Geometry check sheet. Reference: drawing and pictorial views, mm from the part's lowest x, y, z. Coordinates: 2 decimals unless noted, no trailing zeros. Loops run counter-clockwise (first coordinate to the right, second up) from the corner with the lowest first, then second, coordinate; pieces in that order, holes last. Notation, with made-up numbers: M -33.75,-31.5 L -20.75,-31.5 A7 ccw -20.75,-20.5 Z; hole C 50,-39 d3. An arc over 180 degrees is marked long. Write each question's results on one line, items separated by ' | '. Start each with the question number.
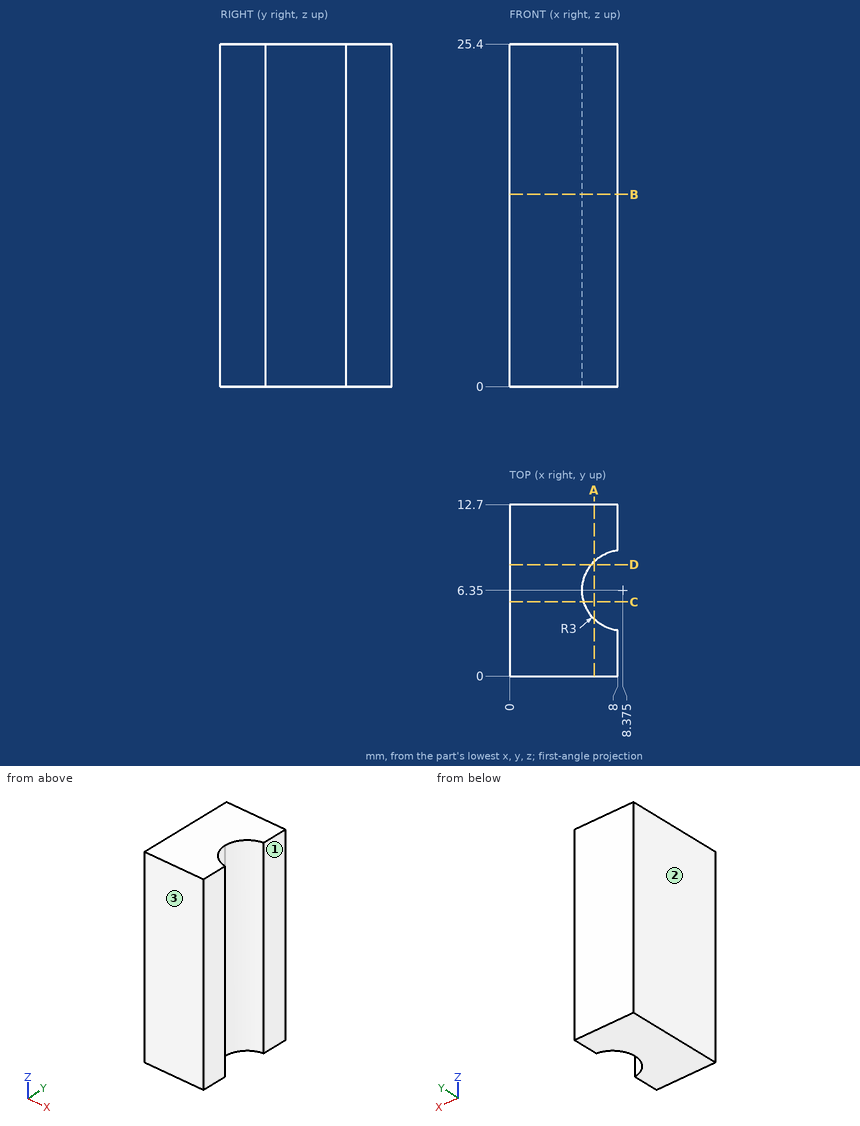
1) Section check B-B (z = 14.25). Enter the section's corners in (x, y) (3 decimals).
2) Section check D-D (y = 8.25). Enter the section's corners in (x, z), then the cut area to 3 significant figures.
3) Section check C-C (y = 5.5). Enter the section's corners in (x, z).
4) Release check for a two-part mould opening along X. For the marked faces 1, 2 and 3 record: +X half, -X half, draft (parallel to the pull), parting line (faces both ways), or undercut.
5) Thickness scan on probe 1 along Y at (x, z) = (7, 15); probe 2 along Y at (x, z) = (6, 18.75); probe 3 along X at (y, z) = (6.75, 5). Record the ranges inside material, lowest first.
6) Section check A-A (x = 6.25). Enter the section's corners in (y, z).
Return value:
1) outline: M 0,0 L 8,0 L 8,3.374 A3 cw 5.375,6.35 A3 cw 8,9.326 L 8,12.7 L 0,12.7 Z
2) outline: M 0,0 L 6.05,0 L 6.05,25.4 L 0,25.4 Z | area: 154 mm2
3) outline: M 0,0 L 5.5,0 L 5.5,25.4 L 0,25.4 Z
4) face 1: +X half | face 2: -X half | face 3: draft
5) probe 1: y = 0 to 3.68, 9.02 to 12.7 | probe 2: y = 0 to 4.52, 8.18 to 12.7 | probe 3: x = 0 to 5.4
6) outline: M 0,0 L 4.23,0 L 4.23,25.4 L 0,25.4 Z; M 8.47,0 L 12.7,0 L 12.7,25.4 L 8.47,25.4 Z
